Work out the finished part from the listing and answer in its coordinate system (mm). Face numbers are marked on the shaded views. A direction names the side the tool comes from. Coordinates: 2 decimals unless noted, no trailing zeros. Order: outer loops, then holes, each group sorted by start corner. A loop starts at its lowest first (then second) coordinate and runs counter-clockwise, first axis right, second up. Notation, with made-up numbers: M -13.75,-7 L 22.25,-7 A21 ccw 22.25,32 Z; hole C -12,56 d8. An arc over 180 degrees is marked long. Use a Markdown table: item, result. Add a question column.
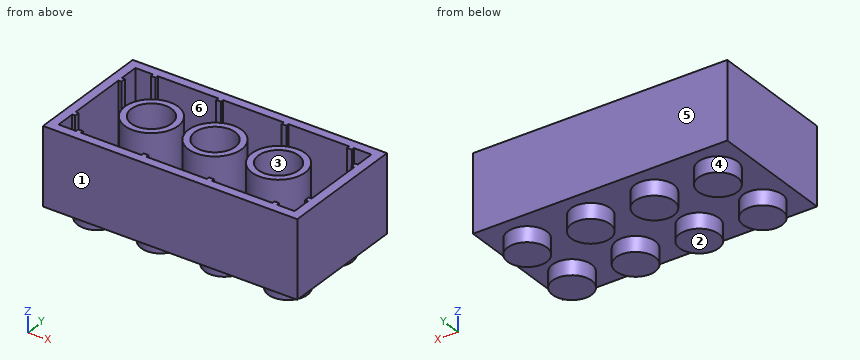
from build123d import *

# Parameters (mm, degrees)
F0_W     = 31.5
F0_H     = 15.75
F0_W_2   = 0.37
F0_H_2   = 0.6
F0_W_3   = 0.6
F0_H_3   = 0.37
F1_DEPTH = 9.55
F0_R     = 3.3
F0_R_2   = 2.5
F2_DEPTH = 1.55
F3_R     = 2.425
F4_DEPTH = 1.9


# Not quite as in the source:
# - a feature names something its author has since deleted; it is built from what else it names


with BuildPart() as f1:
    # F0 (on Top) → F1 (new body)
    with BuildSketch(Plane.XY):
        with Locations((-15.75, 7.875)):
            Rectangle(F0_W, F0_H)
        Polygon((-30.37, 12.225), (-30.37, 14.62), (-28.2, 14.62), (-27.6, 14.62), (-20.1, 14.62), (-19.5, 14.62), (-12, 14.62), (-11.4, 14.62), (-3.9, 14.62), (-3.3, 14.62), (-1.13, 14.62), (-1.13, 12.225), (-1.13, 11.625), (-1.13, 4.125), (-1.13, 3.525), (-1.13, 1.13), (-3.3, 1.13), (-3.9, 1.13), (-11.4, 1.13), (-12, 1.13), (-19.5, 1.13), (-20.1, 1.13), (-27.6, 1.13), (-28.2, 1.13), (-30.37, 1.13), (-30.37, 3.525), (-30.37, 4.125), (-30.37, 11.625), align=None, mode=Mode.SUBTRACT)
        with Locations((-30.185, 11.925)):
            Rectangle(F0_W_2, F0_H_2)
        with Locations((-27.9, 14.435)):
            Rectangle(F0_W_3, F0_H_3)
        with Locations((-19.8, 14.435)):
            Rectangle(F0_W_3, F0_H_3)
        with Locations((-11.7, 14.435)):
            Rectangle(F0_W_3, F0_H_3)
        with Locations((-3.6, 14.435)):
            Rectangle(F0_W_3, F0_H_3)
        with Locations((-1.315, 11.925)):
            Rectangle(F0_W_2, F0_H_2)
        with Locations((-1.315, 3.825)):
            Rectangle(F0_W_2, F0_H_2)
        with Locations((-3.6, 1.315)):
            Rectangle(F0_W_3, F0_H_3)
        with Locations((-11.7, 1.315)):
            Rectangle(F0_W_3, F0_H_3)
        with Locations((-19.8, 1.315)):
            Rectangle(F0_W_3, F0_H_3)
        with Locations((-27.9, 1.315)):
            Rectangle(F0_W_3, F0_H_3)
        with Locations((-30.185, 3.825)):
            Rectangle(F0_W_2, F0_H_2)
    extrude(amount=F1_DEPTH)



with BuildPart() as f1b:
    # F0 (on Top) → F1, piece 2 (new body)
    with BuildSketch(Plane.XY):
        with Locations((-23.625, 7.875)):
            Circle(F0_R)
        with Locations((-23.625, 7.875)):
            Circle(F0_R_2, mode=Mode.SUBTRACT)
    extrude(amount=F1_DEPTH)


with BuildPart() as f1c:
    # F0 (on Top) → F1, piece 3 (new body)
    with BuildSketch(Plane.XY):
        with Locations((-7.875, 7.875)):
            Circle(F0_R)
        with Locations((-7.875, 7.875)):
            Circle(F0_R_2, mode=Mode.SUBTRACT)
    extrude(amount=F1_DEPTH)


with BuildPart() as f1d:
    # F0 (on Top) → F1, piece 4 (new body)
    with BuildSketch(Plane.XY):
        with Locations((-15.75, 7.875)):
            Circle(F0_R)
        with Locations((-15.75, 7.875)):
            Circle(F0_R_2, mode=Mode.SUBTRACT)
    extrude(amount=F1_DEPTH)


with BuildPart() as f1_1:
    add(f1.part)

    add(f1b.part)  # F2 merges F1b

    add(f1c.part)  # F2 merges F1c

    add(f1d.part)  # F2 merges F1d
    # F0 (on Top) → F2 (join)
    with BuildSketch(Plane.XY):
        Polygon((-28.2, 14.62), (-30.37, 14.62), (-30.37, 12.225), (-30, 12.225), (-30, 11.625), (-30.37, 11.625), (-30.37, 4.125), (-30, 4.125), (-30, 3.525), (-30.37, 3.525), (-30.37, 1.13), (-28.2, 1.13), (-28.2, 1.5), (-27.6, 1.5), (-27.6, 1.13), (-20.1, 1.13), (-20.1, 1.5), (-19.5, 1.5), (-19.5, 1.13), (-12, 1.13), (-12, 1.5), (-11.4, 1.5), (-11.4, 1.13), (-3.9, 1.13), (-3.9, 1.5), (-3.3, 1.5), (-3.3, 1.13), (-1.13, 1.13), (-1.13, 3.525), (-1.5, 3.525), (-1.5, 4.125), (-1.13, 4.125), (-1.13, 11.625), (-1.5, 11.625), (-1.5, 12.225), (-1.13, 12.225), (-1.13, 14.62), (-3.3, 14.62), (-3.3, 14.25), (-3.9, 14.25), (-3.9, 14.62), (-11.4, 14.62), (-11.4, 14.25), (-12, 14.25), (-12, 14.62), (-19.5, 14.62), (-19.5, 14.25), (-20.1, 14.25), (-20.1, 14.62), (-27.6, 14.62), (-27.6, 14.25), (-28.2, 14.25), align=None)
        with Locations((-23.625, 7.875)):
            Circle(F0_R, mode=Mode.SUBTRACT)
        with Locations((-15.75, 7.875)):
            Circle(F0_R, mode=Mode.SUBTRACT)
        with Locations((-7.875, 7.875)):
            Circle(F0_R, mode=Mode.SUBTRACT)
        with Locations((-23.625, 7.875)):
            Circle(F0_R_2)
        with Locations((-7.875, 7.875)):
            Circle(F0_R_2)
        with Locations((-15.75, 7.875)):
            Circle(F0_R_2)
    extrude(amount=F2_DEPTH)

    # F3 (on face) → F4 (join)
    with BuildSketch(Plane.XY):
        with Locations((-27.5625, 3.9375)):
            Circle(F3_R)
        with Locations((-11.8125, 3.9375)):
            Circle(F3_R)
        with Locations((-3.9375, 3.9375)):
            Circle(F3_R)
        with Locations((-3.9375, 11.8125)):
            Circle(F3_R)
        with Locations((-11.8125, 11.8125)):
            Circle(F3_R)
        with Locations((-19.6875, 11.8125)):
            Circle(F3_R)
        with Locations((-27.5625, 11.8125)):
            Circle(F3_R)
        with Locations((-19.6875, 3.9375)):
            Circle(F3_R)
    extrude(amount=-F4_DEPTH)


solid = f1_1.part
(1) A cutting plane is placed at B-B on y = 13. Write down the section's boundary in (x, z).
(2) Straight lines are drawn through the part: line 1 (Y direction, x = -15.75, z = 7) (3 decimals); line 2 (X direction, y = 4.75, z = -0.25); line 3 (X direction, y = 2.25, z = 2.25). For each, find the intervals that lie inside material, in ascending order.
(3) The mould has two halves that part along Y. Classify the marked faces 1, 2 and 3: pulls with the +Y half, pulls with the -Y half, needs draft (parallel to the pull), parting line crosses it, or undercut.
(4) A cutting plane is placed at C-C on x = -15.75. Write down the section's boundary in (y, z) (3 decimals), plus the area to 3 significant figures.
(5) A cutting plane is placed at A-A on z = -0.75. Count the separate pieces of the cut face and the enclosed holes in it, plus the area to 3 significant figures.
(6) Which of the six approach directions +Z, -Z, +X, -X, +Y, -Y give full straight-line access (tool end or side, diameter ignored) to the marked faces 4, 5 and 6?
From the geometry:
| question | item | result |
|---|---|---|
| 1 | outline | M -31.5,0 L -29.68,0 L -29.68,-1.9 L -25.45,-1.9 L -25.45,0 L -21.8,0 L -21.8,-1.9 L -17.57,-1.9 L -17.57,0 L -13.93,0 L -13.93,-1.9 L -9.7,-1.9 L -9.7,0 L -6.05,0 L -6.05,-1.9 L -1.82,-1.9 L -1.82,0 L 0,0 L 0,9.55 L -1.13,9.55 L -1.13,1.55 L -30.37,1.55 L -30.37,9.55 L -31.5,9.55 Z |
| 2 | line 1 | y = 0 to 1.13, 4.575 to 5.375, 10.375 to 11.175, 14.62 to 15.75 |
| 2 | line 2 | x = -29.85 to -25.28, -21.97 to -17.4, -14.1 to -9.53, -6.22 to -1.65 |
| 2 | line 3 | x = -31.5 to -30.37, -1.13 to 0 |
| 3 | face 1 | pulls with the -Y half |
| 3 | face 2 | needs draft |
| 3 | face 3 | undercut |
| 4 | outline | M 0,0 L 15.75,0 L 15.75,9.55 L 14.62,9.55 L 14.62,1.55 L 11.175,1.55 L 11.175,9.55 L 10.375,9.55 L 10.375,1.55 L 5.375,1.55 L 5.375,9.55 L 4.575,9.55 L 4.575,1.55 L 1.13,1.55 L 1.13,9.55 L 0,9.55 Z |
| 4 | area | 55.3 mm2 |
| 5 | separate pieces | 8 |
| 5 | enclosed holes | 0 |
| 5 | area | 148 mm2 |
| 6 | face 4 | -Z |
| 6 | face 5 | +Z, -Z, +X, -X, +Y |
| 6 | face 6 | +Z |
